Read the model definition and answer for the solid it produces. Units are mm, in the model's axes. Coordinates: 2 decimals unless noted, no trailing zeros. Write each loop counter-clockwise with the first axis right and the second up, starting at its lowest first coordinate (ties: lowest second). Pieces come first, ordered by that corner, then holes. Notation, with made-up numbers: (43.25, 50) - (59.25, 50) arc R12 ccw to (59.25, 72) - close; hole circle Ø8 at (73.25, 9). An arc over 180 degrees is marked (long way). Use a Markdown table: item, result.
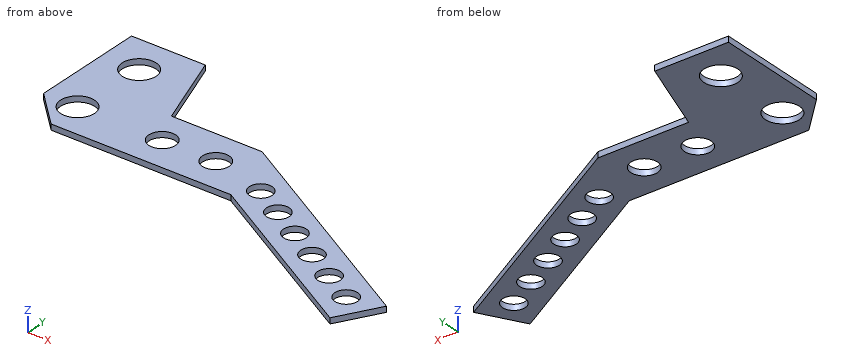
from build123d import *

# Parameters (mm, degrees)
SKETCH2_R           = 6.35
SKETCH2_R_2         = 7.5
SKETCH2_R_3         = 9.525
BOSS_EXTRUDE1_DEPTH = 3.175


with BuildPart() as part:
    # Sketch2 → Boss-Extrude1 (new body)
    with BuildSketch(Plane.XY):
        Polygon((-19.05, 82.55), (22.225, 82.55), (37.775682613, 38.1), (88.575682613, 38.1), (214.73506591, -34.738153907), (201.24131591, -58.110014492), (100.591818382, 0), (0, 0), (-19.05, 19.05), align=None)
        with Locations((109.151133068, 10.639517751)):
            Circle(SKETCH2_R, mode=Mode.SUBTRACT)
        with Locations((126.471641144, 0.639517751)):
            Circle(SKETCH2_R, mode=Mode.SUBTRACT)
        with Locations((143.79214922, -9.360482249)):
            Circle(SKETCH2_R, mode=Mode.SUBTRACT)
        with Locations((161.112657295, -19.360482249)):
            Circle(SKETCH2_R, mode=Mode.SUBTRACT)
        with Locations((178.433165371, -29.360482249)):
            Circle(SKETCH2_R, mode=Mode.SUBTRACT)
        with Locations((195.753673447, -39.360482249)):
            Circle(SKETCH2_R, mode=Mode.SUBTRACT)
        with Locations((47.415438379, 19.05)):
            Circle(SKETCH2_R_2, mode=Mode.SUBTRACT)
        with Locations((77.415438379, 19.05)):
            Circle(SKETCH2_R_2, mode=Mode.SUBTRACT)
        with Locations((0, 19.05)):
            Circle(SKETCH2_R_3, mode=Mode.SUBTRACT)
        with Locations((1.5875, 61.446195183)):
            Circle(SKETCH2_R_3, mode=Mode.SUBTRACT)
    extrude(amount=BOSS_EXTRUDE1_DEPTH)


solid = part.part
(1) A cutting plane is placed at D-D, the plane z = 0.5. Count the separate pieces of the cut face and the enclosed holes in it, and give its area (3 significant figures).
Report:
| item | result |
|---|---|
| separate pieces | 1 |
| enclosed holes | 10 |
| area | 8,180 mm² |
(2) A cutting plane is placed at A-A, the plane x = 73. Write down the section's boundary in (y, z) (1 decimal), and give its area (3 significant figures).
Report:
| item | result |
|---|---|
| outline | (0, 0) - (13, 0) - (13, 3.2) - (0, 3.2) - close; (25.1, 0) - (38.1, 0) - (38.1, 3.2) - (25.1, 3.2) - close |
| area | 82.5 mm² |
(3) This flat-tipped pin is pushed along its axis until it touches: P1, Ø1.5, axis at y = -32, z = 2, coming from the +X side. Where does it stop, or does it pass through?
Report:
| item | result |
|---|---|
| P1 | stops at x = 211.29 |
(4) A cutting plane is placed at C-C, the plane y = 68. Write down the section's boundary in (x, z) (3 decimals), and give its area (3 significant figures).
Report:
| item | result |
|---|---|
| outline | (-19.05, 0) - (-5.324, 0) - (-5.324, 3.175) - (-19.05, 3.175) - close; (8.499, 0) - (27.315, 0) - (27.315, 3.175) - (8.499, 3.175) - close |
| area | 103 mm² |
(5) A cutting plane is placed at B-B, the plane x = -4.5. Write down the section's boundary in (y, z) (3 decimals).
Report:
| item | result |
|---|---|
| outline | (4.5, 0) - (10.655, 0) - (10.655, 3.175) - (4.5, 3.175) - close; (27.445, 0) - (54.12, 0) - (54.12, 3.175) - (27.445, 3.175) - close; (68.772, 0) - (82.55, 0) - (82.55, 3.175) - (68.772, 3.175) - close |
(6) Straight lines are drawn through the part: L1, parallel to X at y = 14, z = 1.5; L2, parallel to Y at x = 0, z = 1.6 (3 decimals); L3, parallel to X at y = -34, z = 2.1. For each, find the intervals that lie inside material, in ascending order.
Report:
| item | result |
|---|---|
| L1 | x = -14 to -8.08, 8.08 to 41.87, 52.96 to 71.87, 82.96 to 103.76, 114.54 to 130.32 |
| L2 | y = 0 to 9.525, 28.575 to 52.054, 70.838 to 82.55 |
| L3 | x = 159.48 to 174.1, 182.77 to 192.35, 199.16 to 213.46 |
